Design review of the part shown in the three views and the two pictorial views. Dimensions are in mm from the part's minimum x, y and z. A direction names the side the tool comes from. Coordinates: 2 decimals unless noted, no trailing zeros. Loops run counter-clockwise (first coordinate to the right, second up) from the corner with the lowest first, then second, coordinate; pieces in that order, holes last. Notation, with made-up numbers: M 59.5,21 L 117.5,21 A31 ccw 117.5,58 Z; hole C 25.25,-11.5 d9. An arc over 180 degrees is marked long. Write item = value, one per line. Start each with the question number.
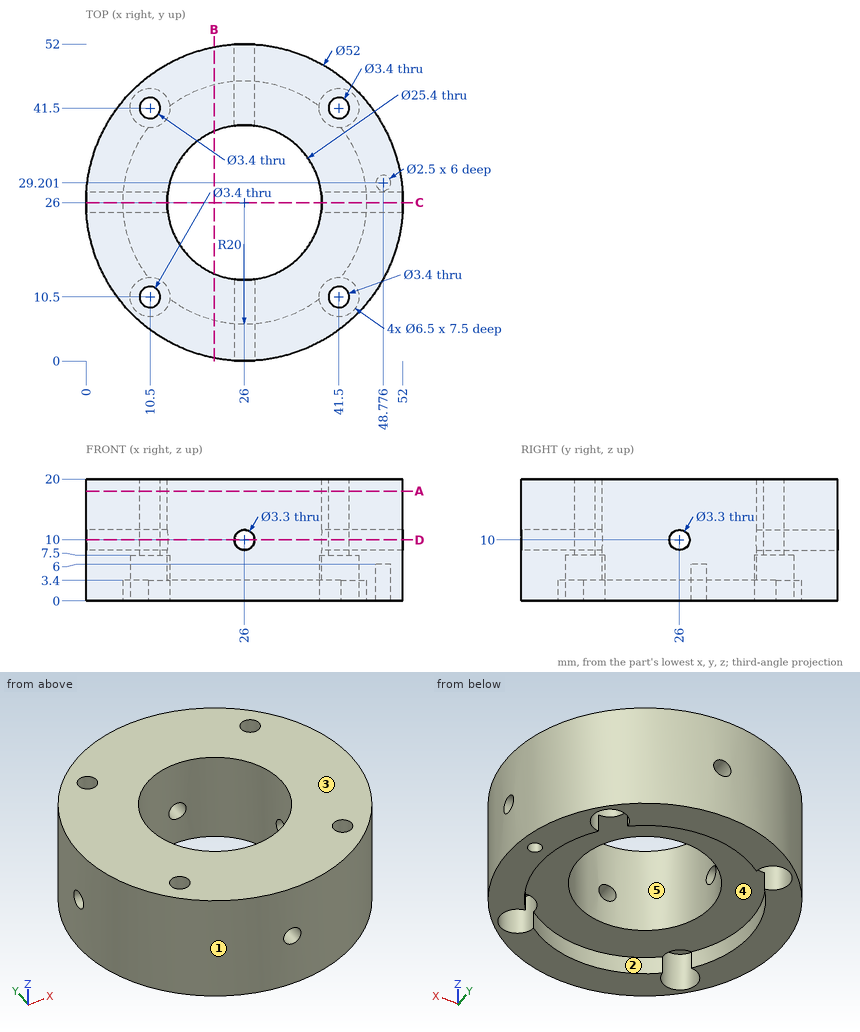
(1) To check wall thickness, follow L1, parallel to Y at x = 11, z = 14.75 (1 decimal); L2, parallel to Y at x = 10.5, z = 16.75 (1 decimal); L3, parallel to X at y = 12, z = 12.75. State the ranges of each line that lie inside material, in increasing order.
(2) Take a section at B-B (x = 21). State the section outline as (y, z) points (1 decimal).
(3) Insertion check: pin 1 (1.5 mm diameter, centred on y = 8, z = 14, fed in from -X); pin 2 (12 mm diameter, centred on x = 45, z = 7.5, fed in from +Y); pin 3 (2 mm diameter, centred on x = 48.5, y = 29.5, fed in from -Z); pin 4 (10 mm diameter, centred on x = 15, z = 18, fed in from +Y). Each pin has a flat end and moves straight along its axis. Give the tip position at first contact, or say it passes through.
(4) Mouldability with a two-part tool opening along X and no side actions: class the marked faces 1, 2 and 3 as +X half, -X half, draft (parallel to the pull), parting line (faces both ways), or undercut.
(5) Take a section at C-C (y = 26). State the section outline as (x, z) points, plus the area to 3 significant figures.
(6) Take a section at A-A (z = 18). State the section outline as (x, y) points.
(7) Take a section at D-D (z = 10). State the section outline as (x, y) points.
(8) Tool access review of the marked faces 4 and 5: name each direction out of +Z, -Z, +X, -X, +Y, -Y from which nothing blocks a thin tool from reaching the whole face with its end or side.
Results list:
q1.L1 = 4.8 to 8.9, 12.1 to 39.9, 43.1 to 47.2
q1.L2 = 5.1 to 8.8, 12.2 to 39.8, 43.2 to 46.9
q1.L3 = 4.09 to 9.7, 11.3 to 40.7, 42.3 to 47.91
q2.outline = M 0.5,0 L 6.6,0 L 6.6,3.4 L 14.3,3.4 L 14.3,20 L 0.5,20 Z; M 37.7,3.4 L 45.4,3.4 L 45.4,0 L 51.5,0 L 51.5,20 L 37.7,20 Z
q3.pin_1 = 6.55
q3.pin_2 = 48.52
q3.pin_3 = 0
q3.pin_4 = 51.3
q4.face_1 = parting line
q4.face_2 = undercut
q4.face_3 = draft
q5.outline = M 0,0 L 6,0 L 6,3.4 L 13.3,3.4 L 13.3,8.35 L 0,8.35 Z; M 0,11.65 L 13.3,11.65 L 13.3,20 L 0,20 Z; M 38.7,3.4 L 46,3.4 L 46,0 L 52,0 L 52,8.35 L 38.7,8.35 Z; M 38.7,11.65 L 52,11.65 L 52,20 L 38.7,20 Z
q5.area = 395 mm^2
q6.outline = C 26,26 d52; hole C 10.5,10.5 d3.4; hole C 10.5,41.5 d3.4; hole C 26,26 d25.4; hole C 41.5,10.5 d3.4; hole C 41.5,41.5 d3.4
q7.outline = M 0.05,24.35 A26 ccw 24.35,0.05 L 24.35,13.41 A12.7 cw 13.41,24.35 Z; M 0.05,27.65 L 13.41,27.65 A12.7 cw 24.35,38.59 L 24.35,51.95 A26 ccw Z; M 27.65,0.05 A26 ccw 51.95,24.35 L 38.59,24.35 A12.7 cw 27.65,13.41 Z; M 27.65,38.59 A12.7 cw 38.59,27.65 L 51.95,27.65 A26 ccw 27.65,51.95 Z; hole C 10.5,10.5 d3.4; hole C 10.5,41.5 d3.4; hole C 41.5,10.5 d3.4; hole C 41.5,41.5 d3.4
q8.face_4 = -Z
q8.face_5 = +Z, -Z
